```python
from build123d import *

# Parameters (mm, degrees)
SKETCH1_W                                      = 539
SKETCH1_H                                      = 299
BOSS_EXTRUDE1_DEPTH                            = 3
SKETCH2_W                                      = 20
SKETCH2_H                                      = 51
CUT_EXTRUDE1_DEPTH                             = 309.203666429
CSK_FOR_M3_FLAT_HEAD_MACHINE_SCREW1_AT_2_COUNT = 2
CSK_FOR_M3_FLAT_HEAD_MACHINE_SCREW1_AT_2_PITCH = 50.429256866
CSK_FOR_M3_FLAT_HEAD_MACHINE_SCREW1_AT_3_COUNT = 2
CSK_FOR_M3_FLAT_HEAD_MACHINE_SCREW1_AT_3_PITCH = 94.539771311
CSK_FOR_M3_FLAT_HEAD_MACHINE_SCREW1_AT_4_COUNT = 2
CSK_FOR_M3_FLAT_HEAD_MACHINE_SCREW1_AT_4_PITCH = 141.314201671
CSK_FOR_M3_FLAT_HEAD_MACHINE_SCREW1_AT_5_COUNT = 2
CSK_FOR_M3_FLAT_HEAD_MACHINE_SCREW1_AT_5_PITCH = 188.996190438
CSK_FOR_M3_FLAT_HEAD_MACHINE_SCREW1_AT_6_COUNT = 2
CSK_FOR_M3_FLAT_HEAD_MACHINE_SCREW1_AT_6_PITCH = 236.347731108
CUT_EXTRUDE3_DEPTH                             = 309.203666429
CUT_EXTRUDE3_DEPTH_BACK                        = 309.203666429
SKETCH6_W                                      = 70
SKETCH6_H                                      = 20
SKETCH9_W                                      = 60
SKETCH9_H                                      = 60
CUT_EXTRUDE4_DEPTH                             = 309.203666429
FILLET1_R                                      = 0.5


with BuildPart() as part:
    # Sketch1 → Boss-Extrude1 (new body)
    with BuildSketch(Plane(origin=(0, 0, 0), x_dir=(1, 0, 0), z_dir=(0, 1, 0))):
        Rectangle(SKETCH1_W, SKETCH1_H)
    extrude(amount=BOSS_EXTRUDE1_DEPTH)

    # Sketch2 → Cut-Extrude1 (cut, through all)
    with BuildSketch(Plane(origin=(0, 3, 0), x_dir=(1, 0, 0), z_dir=(0, 1, 0))):
        with Locations((-259.5, 0)):
            Rectangle(SKETCH2_W, SKETCH2_H)
    cut_extrude1 = extrude(amount=-CUT_EXTRUDE1_DEPTH, mode=Mode.SUBTRACT)

    # Mirror1: Cut-Extrude1 across plane
    add(cut_extrude1.mirror(Plane(origin=(0, 0, 0), x_dir=(0, 0, 1), z_dir=(1, 0, 0))), mode=Mode.SUBTRACT)

    # Sketch4 → CSK for M3 Flat Head Machine Screw1 (revolve, cut)
    with BuildSketch(Plane(origin=(-257.5, 3, 45), x_dir=(0, 0, 1), z_dir=(1, 0, 0))):
        Polygon((0, 0), (0, 3), (1.6, 3), (1.6, 1.55), (3.15, 0), align=None)
    csk_for_m3_flat_head_machine_screw1 = revolve(axis=Axis((-257.5, 9.35, 45), (0, -1, 0)), mode=Mode.SUBTRACT)

    # CSK for M3 Flat Head Machine Screw1 at 2: CSK for M3 Flat Head Machine Screw1 ×2
    with Locations(*[Vector(0.9339816393782528, 0, -0.357321000368452) * (i * CSK_FOR_M3_FLAT_HEAD_MACHINE_SCREW1_AT_2_PITCH) for i in range(1, CSK_FOR_M3_FLAT_HEAD_MACHINE_SCREW1_AT_2_COUNT)]):
        add(csk_for_m3_flat_head_machine_screw1, mode=Mode.SUBTRACT)

    # CSK for M3 Flat Head Machine Screw1 at 3: CSK for M3 Flat Head Machine Screw1 ×2
    with Locations(*[Vector(0.9964060489398768, 0, -0.0847052869425741) * (i * CSK_FOR_M3_FLAT_HEAD_MACHINE_SCREW1_AT_3_PITCH) for i in range(1, CSK_FOR_M3_FLAT_HEAD_MACHINE_SCREW1_AT_3_COUNT)]):
        add(csk_for_m3_flat_head_machine_screw1, mode=Mode.SUBTRACT)

    # CSK for M3 Flat Head Machine Screw1 at 4: CSK for M3 Flat Head Machine Screw1 ×2
    with Locations(*[Vector(0.9998995028746508, 0, 0.01417688791753526) * (i * CSK_FOR_M3_FLAT_HEAD_MACHINE_SCREW1_AT_4_PITCH) for i in range(1, CSK_FOR_M3_FLAT_HEAD_MACHINE_SCREW1_AT_4_COUNT)]):
        add(csk_for_m3_flat_head_machine_screw1, mode=Mode.SUBTRACT)

    # CSK for M3 Flat Head Machine Screw1 at 5: CSK for M3 Flat Head Machine Screw1 ×2
    with Locations(*[Vector(0.9968454896555541, 0, 0.07936667911270336) * (i * CSK_FOR_M3_FLAT_HEAD_MACHINE_SCREW1_AT_5_PITCH) for i in range(1, CSK_FOR_M3_FLAT_HEAD_MACHINE_SCREW1_AT_5_COUNT)]):
        add(csk_for_m3_flat_head_machine_screw1, mode=Mode.SUBTRACT)

    # CSK for M3 Flat Head Machine Screw1 at 6: CSK for M3 Flat Head Machine Screw1 ×2
    with Locations(*[Vector(0.9964132039506463, 0, 0.08462107889177463) * (i * CSK_FOR_M3_FLAT_HEAD_MACHINE_SCREW1_AT_6_PITCH) for i in range(1, CSK_FOR_M3_FLAT_HEAD_MACHINE_SCREW1_AT_6_COUNT)]):
        add(csk_for_m3_flat_head_machine_screw1, mode=Mode.SUBTRACT)

    # Sketch6 → Cut-Extrude3 (cut, two sides: drawn at the far end of the back side and taken through both)
    with BuildSketch(Plane(origin=(0, 3, 0), x_dir=(1, 0, 0), z_dir=(0, 1, 0)).offset(-CUT_EXTRUDE3_DEPTH_BACK)):
        Polygon((199.5, 149.5), (199.5, 129.5), (249.5, 129.5), (249.5, 91.5), (269.5, 91.5), (269.5, 149.5), align=None)
        with Locations((234.5, -139.5)):
            Rectangle(SKETCH6_W, SKETCH6_H)
    extrude(amount=CUT_EXTRUDE3_DEPTH + CUT_EXTRUDE3_DEPTH_BACK, mode=Mode.SUBTRACT)

    # Mirror2: CSK for M3 Flat Head Machine Screw1 across plane
    add(csk_for_m3_flat_head_machine_screw1.mirror(Plane(origin=(0, 0, 0), x_dir=(0, 0, 1), z_dir=(1, 0, 0))), mode=Mode.SUBTRACT)

    # Mirror2 copy 1 sketch → Mirror2 copy 1 (revolve, cut)
    with BuildSketch(Plane(origin=(210.4, 3, 26.980567489), x_dir=(0, 0, 1), z_dir=(-1, 0, 0))):
        Polygon((0, 0), (0, -3), (1.6, -3), (1.6, -1.55), (3.15, 0), align=None)
    revolve(axis=Axis((210.4, 9.35, 26.980567489), (0, 1, 0)), mode=Mode.SUBTRACT)

    # Mirror2 copy 2 sketch → Mirror2 copy 2 (revolve, cut)
    with BuildSketch(Plane(origin=(163.3, 3, 36.991981544), x_dir=(0, 0, 1), z_dir=(-1, 0, 0))):
        Polygon((0, 0), (0, -3), (1.6, -3), (1.6, -1.55), (3.15, 0), align=None)
    revolve(axis=Axis((163.3, 9.35, 36.991981544), (0, 1, 0)), mode=Mode.SUBTRACT)

    # Mirror2 copy 3 sketch → Mirror2 copy 3 (revolve, cut)
    with BuildSketch(Plane(origin=(116.2, 3, 47.003395598), x_dir=(0, 0, 1), z_dir=(-1, 0, 0))):
        Polygon((0, 0), (0, -3), (1.6, -3), (1.6, -1.55), (3.15, 0), align=None)
    revolve(axis=Axis((116.2, 9.35, 47.003395598), (0, 1, 0)), mode=Mode.SUBTRACT)

    # Mirror2 copy 4 sketch → Mirror2 copy 4 (revolve, cut)
    with BuildSketch(Plane(origin=(69.1, 3, 60), x_dir=(0, 0, 1), z_dir=(-1, 0, 0))):
        Polygon((0, 0), (0, -3), (1.6, -3), (1.6, -1.55), (3.15, 0), align=None)
    revolve(axis=Axis((69.1, 9.35, 60), (0, 1, 0)), mode=Mode.SUBTRACT)

    # Mirror2 copy 5 sketch → Mirror2 copy 5 (revolve, cut)
    with BuildSketch(Plane(origin=(22, 3, 65), x_dir=(0, 0, 1), z_dir=(-1, 0, 0))):
        Polygon((0, 0), (0, -3), (1.6, -3), (1.6, -1.55), (3.15, 0), align=None)
    revolve(axis=Axis((22, 9.35, 65), (0, 1, 0)), mode=Mode.SUBTRACT)

    # Mirror3: CSK for M3 Flat Head Machine Screw1 across plane
    add(csk_for_m3_flat_head_machine_screw1.mirror(Plane.XY), mode=Mode.SUBTRACT)

    # Mirror3 copy 1 sketch → Mirror3 copy 1 (revolve, cut)
    with BuildSketch(Plane(origin=(-210.4, 3, -26.980567489), x_dir=(0, 0, -1), z_dir=(1, 0, 0))):
        Polygon((0, 0), (0, -3), (1.6, -3), (1.6, -1.55), (3.15, 0), align=None)
    revolve(axis=Axis((-210.4, 9.35, -26.980567489), (0, 1, 0)), mode=Mode.SUBTRACT)

    # Mirror3 copy 2 sketch → Mirror3 copy 2 (revolve, cut)
    with BuildSketch(Plane(origin=(-163.3, 3, -36.991981544), x_dir=(0, 0, -1), z_dir=(1, 0, 0))):
        Polygon((0, 0), (0, -3), (1.6, -3), (1.6, -1.55), (3.15, 0), align=None)
    revolve(axis=Axis((-163.3, 9.35, -36.991981544), (0, 1, 0)), mode=Mode.SUBTRACT)

    # Mirror3 copy 3 sketch → Mirror3 copy 3 (revolve, cut)
    with BuildSketch(Plane(origin=(-116.2, 3, -47.003395598), x_dir=(0, 0, -1), z_dir=(1, 0, 0))):
        Polygon((0, 0), (0, -3), (1.6, -3), (1.6, -1.55), (3.15, 0), align=None)
    revolve(axis=Axis((-116.2, 9.35, -47.003395598), (0, 1, 0)), mode=Mode.SUBTRACT)

    # Mirror3 copy 4 sketch → Mirror3 copy 4 (revolve, cut)
    with BuildSketch(Plane(origin=(-69.1, 3, -60), x_dir=(0, 0, -1), z_dir=(1, 0, 0))):
        Polygon((0, 0), (0, -3), (1.6, -3), (1.6, -1.55), (3.15, 0), align=None)
    revolve(axis=Axis((-69.1, 9.35, -60), (0, 1, 0)), mode=Mode.SUBTRACT)

    # Mirror3 copy 5 sketch → Mirror3 copy 5 (revolve, cut)
    with BuildSketch(Plane(origin=(-22, 3, -65), x_dir=(0, 0, -1), z_dir=(1, 0, 0))):
        Polygon((0, 0), (0, -3), (1.6, -3), (1.6, -1.55), (3.15, 0), align=None)
    revolve(axis=Axis((-22, 9.35, -65), (0, 1, 0)), mode=Mode.SUBTRACT)

    # Mirror3 copy 6 sketch → Mirror3 copy 6 (revolve, cut)
    with BuildSketch(Plane(origin=(257.5, 3, -45), x_dir=(0, 0, -1), z_dir=(-1, 0, 0))):
        Polygon((0, 0), (0, 3), (1.6, 3), (1.6, 1.55), (3.15, 0), align=None)
    revolve(axis=Axis((257.5, 9.35, -45), (0, -1, 0)), mode=Mode.SUBTRACT)

    # Mirror3 copy 7 sketch → Mirror3 copy 7 (revolve, cut)
    with BuildSketch(Plane(origin=(210.4, 3, -26.980567489), x_dir=(0, 0, -1), z_dir=(-1, 0, 0))):
        Polygon((0, 0), (0, 3), (1.6, 3), (1.6, 1.55), (3.15, 0), align=None)
    revolve(axis=Axis((210.4, 9.35, -26.980567489), (0, -1, 0)), mode=Mode.SUBTRACT)

    # Mirror3 copy 8 sketch → Mirror3 copy 8 (revolve, cut)
    with BuildSketch(Plane(origin=(163.3, 3, -36.991981544), x_dir=(0, 0, -1), z_dir=(-1, 0, 0))):
        Polygon((0, 0), (0, 3), (1.6, 3), (1.6, 1.55), (3.15, 0), align=None)
    revolve(axis=Axis((163.3, 9.35, -36.991981544), (0, -1, 0)), mode=Mode.SUBTRACT)

    # Mirror3 copy 9 sketch → Mirror3 copy 9 (revolve, cut)
    with BuildSketch(Plane(origin=(116.2, 3, -47.003395598), x_dir=(0, 0, -1), z_dir=(-1, 0, 0))):
        Polygon((0, 0), (0, 3), (1.6, 3), (1.6, 1.55), (3.15, 0), align=None)
    revolve(axis=Axis((116.2, 9.35, -47.003395598), (0, -1, 0)), mode=Mode.SUBTRACT)

    # Mirror3 copy 10 sketch → Mirror3 copy 10 (revolve, cut)
    with BuildSketch(Plane(origin=(69.1, 3, -60), x_dir=(0, 0, -1), z_dir=(-1, 0, 0))):
        Polygon((0, 0), (0, 3), (1.6, 3), (1.6, 1.55), (3.15, 0), align=None)
    revolve(axis=Axis((69.1, 9.35, -60), (0, -1, 0)), mode=Mode.SUBTRACT)

    # Mirror3 copy 11 sketch → Mirror3 copy 11 (revolve, cut)
    with BuildSketch(Plane(origin=(22, 3, -65), x_dir=(0, 0, -1), z_dir=(-1, 0, 0))):
        Polygon((0, 0), (0, 3), (1.6, 3), (1.6, 1.55), (3.15, 0), align=None)
    revolve(axis=Axis((22, 9.35, -65), (0, -1, 0)), mode=Mode.SUBTRACT)

    # Sketch9 → Cut-Extrude4 (cut, through all)
    with BuildSketch(Plane(origin=(0, 3, 0), x_dir=(1, 0, 0), z_dir=(0, 1, 0))):
        Rectangle(SKETCH9_W, SKETCH9_H)
    extrude(amount=-CUT_EXTRUDE4_DEPTH, mode=Mode.SUBTRACT)

    # Fillet1
    fillet1_edges = [part.edges().sort_by_distance(p)[0] for p in [
        (269.5, 1.5, 129.5),
        (199.5, 1.5, 149.5),
        (199.5, 1.5, 129.5),
        (-269.5, 1.5, 25.5),
        (-269.5, 1.5, -25.5),
        (-249.5, 1.5, -25.5),
        (-249.5, 1.5, 25.5),
        (269.5, 1.5, -25.5),
        (269.5, 1.5, 25.5),
        (249.5, 1.5, 25.5),
        (249.5, 1.5, -25.5),
        (-269.5, 1.5, -149.5),
        (-269.5, 1.5, 149.5),
        (199.5, 1.5, -149.5),
        (269.5, 1.5, -91.5),
        (249.5, 1.5, -91.5),
        (249.5, 1.5, -129.5),
        (199.5, 1.5, -129.5),
    ]]
    fillet(fillet1_edges, radius=FILLET1_R)


solid = part.part
```
Build history of the part. All positions in model axes, mm. Coordinates: 2 decimals unless noted, no trailing zeros. One line per question, with ' | ' between items. Start each with the question number.
1. Flat gauge pins, fed straight in: P1, Ø3.5, axis at x = 116.2, z = 47, coming from the +Y side; P2, Ø4, axis at x = -257.5, z = -45, coming from the +Y side; P3, Ø0.9, axis at x = 261, y = 2, coming from the -Z side. Where does each tip first touch, or does it go through?
2. Cut at A-A (y = 2.3). Count the separate pieces of the cut face and the enclosed holes in it, plus the area to 3 significant figures.
3. Wall check: line 1 along Z through (x, y) = (210.4, 1.05); line 2 along X through (y, z) = (0.9, 60); line 3 along X through (y, z) = (2.35, -3.5). Give the ranges that are in metal, low to high. Write a range as [from, to].
The answers:
1) P1: stops at y = 1.6 | P2: stops at y = 1.85 | P3: stops at z = -91.5
2) separate pieces: 1 | enclosed holes: 25 | area: 152,000 mm2
3) line 1: z = [-129.5, -28.58], [-25.38, 25.38], [28.58, 129.5] | line 2: x = [-269.5, -70.7], [-67.5, 67.5], [70.7, 269.5] | line 3: x = [-249.5, -30], [30, 249.5]
